from build123d import *

# Parameters (mm, degrees)
SKETCH1_R           = 32.5
BOSS_EXTRUDE1_DEPTH = 2
CUT_EXTRUDE1_DEPTH  = 2
SKETCH3_W           = 3
SKETCH3_H           = 6
CUT_EXTRUDE2_DEPTH  = 2
FILLET1_R           = 1
FILLET2_R           = 2
SKETCH4_R           = 1.5
CUT_EXTRUDE3_DEPTH  = 2


with BuildPart() as part:
    # Sketch1 → Boss-Extrude1 (new body)
    with BuildSketch(Plane(origin=(0, 0, 0), x_dir=(1, 0, 0), z_dir=(0, 1, 0))):
        with BuildLine():
            Line((-39.655963303, 26.146788991), (-25, 75))
            Line((-25, 75), (25, 75))
            Line((25, 75), (39.655963303, 26.146788991))
            ThreePointArc((39.655963303, 26.146788991), (47.5, 0), (39.655963303, -26.146788991))
            Line((39.655963303, -26.146788991), (25, -75))
            Line((25, -75), (-25, -75))
            Line((-25, -75), (-39.655963303, -26.146788991))
            ThreePointArc((-39.655963303, -26.146788991), (-47.5, 0), (-39.655963303, 26.146788991))
        make_face()
        with Locations(Location((0, 0, 0), (0, 0, 270))):
            Circle(SKETCH1_R, mode=Mode.SUBTRACT)
    extrude(amount=BOSS_EXTRUDE1_DEPTH)

    # Sketch2 → Cut-Extrude1 (cut)
    with BuildSketch(Plane(origin=(0, 2, 0), x_dir=(1, 0, 0), z_dir=(0, 1, 0))):
        Polygon((41.012193309, 36.769552622), (30.405591591, 26.162950904), (26.162950904, 30.405591591), (36.769552622, 41.012193309), align=None)
        Polygon((-41.012193309, 36.769552622), (-36.769552622, 41.012193309), (-26.162950904, 30.405591591), (-30.405591591, 26.162950904), align=None)
        Polygon((36.769552622, -41.012193309), (26.162950904, -30.405591591), (30.405591591, -26.162950904), (41.012193309, -36.769552622), align=None)
        Polygon((-41.012193309, -36.769552622), (-30.405591591, -26.162950904), (-26.162950904, -30.405591591), (-36.769552622, -41.012193309), align=None)
    extrude(amount=-CUT_EXTRUDE1_DEPTH, mode=Mode.SUBTRACT)

    # Sketch3 → Cut-Extrude2 (cut)
    with BuildSketch(Plane(origin=(0, 2, 0), x_dir=(1, 0, 0), z_dir=(0, 1, 0))):
        with Locations((0, 32.5)):
            Rectangle(SKETCH3_W, SKETCH3_H)
        with Locations((0, -32.5)):
            Rectangle(SKETCH3_W, SKETCH3_H)
    extrude(amount=-CUT_EXTRUDE2_DEPTH, mode=Mode.SUBTRACT)

    # Fillet1
    fillet1_edges = [part.edges().sort_by_distance(p)[0] for p in [
        (-1.5, 1, -32.465366161),
        (1.5, 1, -32.465366161),
        (1.5, 1, -35.5),
        (-1.5, 1, -35.5),
        (1.5, 1, 32.465366161),
        (-1.5, 1, 32.465366161),
        (-1.5, 1, 35.5),
        (1.5, 1, 35.5),
    ]]
    fillet(fillet1_edges, radius=FILLET1_R)

    # Fillet2
    fillet2_edges = [part.edges().sort_by_distance(p)[0] for p in [
        (25, 1, 75),
        (-25, 1, 75),
        (-25, 1, -75),
        (25, 1, -75),
    ]]
    fillet(fillet2_edges, radius=FILLET2_R)

    # Sketch4 → Cut-Extrude3 (cut)
    with BuildSketch(Plane(origin=(0, 2, 0), x_dir=(1, 0, 0), z_dir=(0, 1, 0))):
        with Locations(Location((-17.75, 30.743901834, 0), (0, 0, 270))):
            Circle(SKETCH4_R)
        with Locations(Location((17.75, 30.743901834, 0), (0, 0, 90))):
            Circle(SKETCH4_R)
        with Locations(Location((17.75, -30.743901834, 0), (0, 0, 270))):
            Circle(SKETCH4_R)
        with Locations(Location((-17.75, -30.743901834, 0), (0, 0, 90))):
            Circle(SKETCH4_R)
    extrude(amount=-CUT_EXTRUDE3_DEPTH, mode=Mode.SUBTRACT)


solid = part.part
Work out the finished part from the listing and answer in its coordinate system (mm). A direction names the side the tool comes from. Give positions to 0.01 mm unless a question says otherwise; leave off trailing zeros. Order: outer loops, then holes, each group sorted by start corner. A loop starts at its lowest first (then second) coordinate and runs counter-clockwise, first axis right, second up. Notation, with made-up numbers: (-25.5, -23.5) -> (-9.5, -23.5) arc R19 ccw to (-9.5, -2.5) -> close; hole circle Ø2 at (75.25, -21). An arc over 180 degrees is marked (long way). Answer as a JSON object with one key per item and string values. Group by question number.
1. Section C-C on y = 1.55 is taken. Count the separate pieces of the cut face and the enclosed holes in it, plus the area to 3 significant figures.
2. A tool of negligible diameter and unlimited length cuts with its end or side. For faces 4 (the cylindrical face through (32.493, 0.986, 0.681)), 5 (the flat face through (-30.564, 0.986, -56.452)), from which of +Z, -Z, +X, -X, +Y, -Y can it reach the whole face along a straight path? Write none if from no direction.
3. The mould has two halves that part along X. Classify faces 1 (the cylindrical face through (-32.493, 0.986, -0.681)), 2 (the flat face through (-30.423, 0.986, 56.925)), 3 (the cylindrical face through (47.5, 1, -0.4)): released by +X, released by -X, zero draft, split by the parting line, or undercut.
4. Flat-ended cylindrical pins translate along their axes: pin 1 Ø2.5 at (x, z) = (17.75, 30.74) entering from -Y; pin 2 Ø0.5 at (y, z) = (1, -34) entering from +X; pin 3 Ø0.9 at (y, z) = (1, 34) entering from -X. Find the tip coordinate at first contact, or state that the pin passes through.
5. Consider line 1 along X through (y, z) = (1.25, -33); line 2 along X through (y, z) = (0.5, -0.5); line 3 along X through (y, z) = (0.55, -32.5). Determine where each line is inside the solid, lowest interval first. Write a range as [from, to].
6. Section A-A on z = 12.5 is taken. Determine the outline of the cut face in (x, y), plus the area to 3 significant figures.
7. Section B-B on x = 11 is taken. Determine the outline of the cut face in (y, z), plus the area to 3 significant figures.
8. Section D-D on x = -17.75 is taken. Determine the outline of the cut face in (y, z).
Result sheet:
{
 "1": {"separate pieces": "1", "enclosed holes": "5", "area": "7,380 mm^2"},
 "2": {"face 4": "+Y, -Y", "face 5": "-Z, -X, +Y, -Y"},
 "3": {"face 1": "undercut", "face 2": "released by -X", "face 3": "released by +X"},
 "4": {"pin 1": "passes through", "pin 2": "stops at x = 30.01", "pin 3": "stops at x = -30.21"},
 "5": {"line 1": "x = [-37.6, -37.24], [-28.76, -1.59], [1.59, 28.76], [37.24, 37.6]", "line 2": "x = [-47.5, -32.5], [32.5, 47.5]", "line 3": "x = [-37.75, -36.74], [-28.26, -2.08], [2.08, 28.26], [36.74, 37.75]"},
 "6": {"outline": "(-45.83, 0) -> (-30, 0) -> (-30, 2) -> (-45.83, 2) -> close; (30, 0) -> (45.83, 0) -> (45.83, 2) -> (30, 2) -> close", "area": "63.3 mm^2"},
 "7": {"outline": "(0, -75) -> (2, -75) -> (2, -30.58) -> (0, -30.58) -> close; (0, 30.58) -> (2, 30.58) -> (2, 75) -> (0, 75) -> close", "area": "178 mm^2"},
 "8": {"outline": "(0, -75) -> (2, -75) -> (2, -32.24) -> (0, -32.24) -> close; (0, -29.24) -> (2, -29.24) -> (2, -27.22) -> (0, -27.22) -> close; (0, 27.22) -> (2, 27.22) -> (2, 29.24) -> (0, 29.24) -> close; (0, 32.24) -> (2, 32.24) -> (2, 75) -> (0, 75) -> close"}
}
